The listing builds one solid part. Answer for the finished solid, in the listing's coordinates (mm). Face numbers are marked on the shaded views. Round coordinates to 2 decimals unless told otherwise and drop trailing zeros. Write each loop counter-clockwise with the first axis right and the second up, starting at its lowest first coordinate (ties: lowest second). Pieces come first, ordered by that corner, then holes. Notation, with made-up numbers: M -22.75,51.25 L -11.75,51.25 A17 cw -11.75,62.25 Z; hole C -23,9.5 d10. An arc over 180 degrees is marked long. Write each question's results on one line, items separated by ' | '.
from build123d import *

# Parameters (mm, degrees)
F0_R     = 20
F0_R_2   = 18
F1_DEPTH = 50
F0_R_3   = 22
F2_DEPTH = 55
F3_DEPTH = 40
F4_R     = 0.75
F5_R     = 0.75
F6_R     = 5


with BuildPart() as f1:
    # F0 (on Top) → F1 (new body)
    with BuildSketch(Plane.XY):
        Circle(F0_R)
        Circle(F0_R_2, mode=Mode.SUBTRACT)
        Circle(F0_R_2)
    extrude(amount=F1_DEPTH)

    # F0 (on Top) → F2 (join)
    with BuildSketch(Plane.XY):
        Circle(F0_R_3)
        Circle(F0_R, mode=Mode.SUBTRACT)
    extrude(amount=F2_DEPTH)

    # F0 (on Top) → F3 (cut)
    with BuildSketch(Plane.XY):
        Circle(F0_R_2)
    extrude(amount=F3_DEPTH, mode=Mode.SUBTRACT)

    # F4
    f4_edges = [f1.edges().sort_by_distance(p)[0] for p in [
        (-20, 0, 55),
    ]]
    fillet(f4_edges, radius=F4_R)

    # F5
    f5_edges = [f1.edges().sort_by_distance(p)[0] for p in [
        (-22, 0, 55),
    ]]
    fillet(f5_edges, radius=F5_R)

    # F6
    f6_edges = [f1.edges().sort_by_distance(p)[0] for p in [
        (-18, 0, 40),
    ]]
    fillet(f6_edges, radius=F6_R)


solid = f1.part
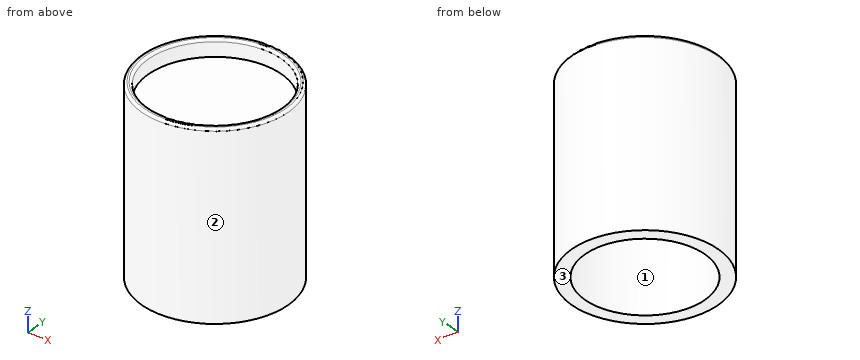
1) The mould has two halves that part along Y. Classify the marked faces 1, 2 and 3: +Y half, -Y half, draft (parallel to the pull), parting line (faces both ways), or undercut.
Return value:
face 1: undercut | face 2: parting line | face 3: draft
2) Each of these flat-tipped pins is pushed along its axis until it touches: pin 1 (1.5 mm diameter, centred on x = 15, z = 41.5, fed in from -Y); pin 2 (3 mm diameter, centred on x = 1.5, y = 7.5, fed in from -Z); pin 3 (1 mm diameter, centred on x = 2.5, z = 32, fed in from +Y). Where does it stop, or does it pass through?
Return value:
pin 1: y = -16.76 | pin 2: z = 40 | pin 3: y = 21.91
3) Section B-B (z = 31.5) is taken. Determine the outline of the cut face in (x, y).
Return value:
outline: C 0,0 d44; hole C 0,0 d36
4) Find the intervals of material crossed by line 1 (Y direction, x = 0, z = 14); line 2 (Y direction, x = 0, z = 53); line 3 (Z direction, x = 8, y = 10), in increasing order.
Return value:
line 1: -22 to -18, 18 to 22 | line 2: -22 to -20, 20 to 22 | line 3: 40 to 50
5) Section A-A (x = 0) is taken. Determine the outline of the cut face in (y, z).
Return value:
outline: M -22,0 L -18,0 L -18,35 A5 cw -13,40 L 13,40 A5 cw 18,35 L 18,0 L 22,0 L 22,54.25 A0.75 ccw 21.25,55 L 20.75,55 A0.75 ccw 20,54.25 L 20,50 L -20,50 L -20,54.25 A0.75 ccw -20.75,55 L -21.25,55 A0.75 ccw -22,54.25 Z
